Here's the drawing with two shaded views (mm, measured from the low corner). I have some questions. Round coordinates to 2 decimals unless told otherwise and drop trailing zeros. Write each loop counter-clockwise with the first axis right and the second up, starting at its lowest first coordinate (ties: lowest second). Pieces come first, ordered by that corner, then holes. Notation, with made-up numbers: (-24, 86) - (28, 86) arc R15 ccw to (28, 103) - close; hole circle Ø11 at (66.5, 79). An arc over 180 degrees is marked (long way). Return JSON: item names as keys, results as strings. Group by question number.
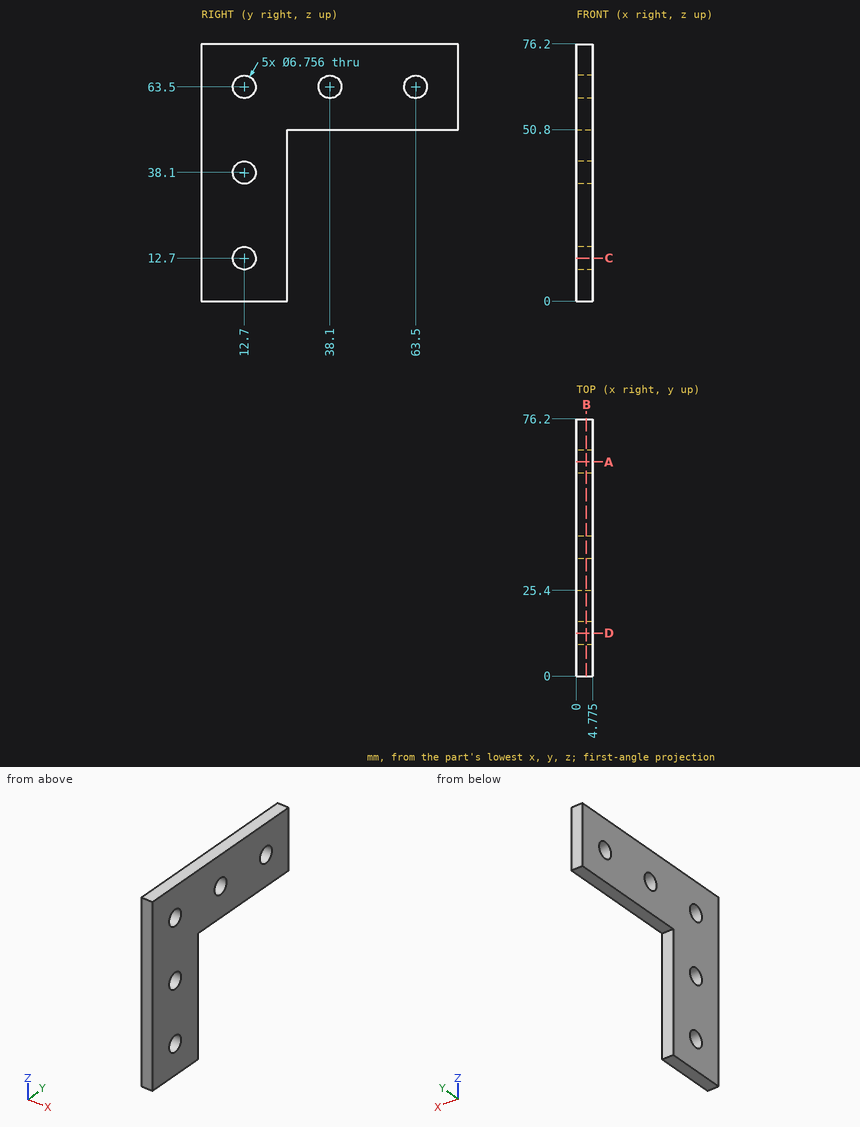
1) Imagine slicing it at A-A (y = 63.5). Please give me the cut outline in (x, z) (1 decimal).
2) Will these pins go through, and if not, where does the flat tip stop? pin 1 Ø1.4 at (x, z) = (1.5, 17.5) entering from +Y; pin 2 Ø6 at (y, z) = (38.1, 63.5) entering from -X; pin 3 Ø2 at (x, y) = (3.5, 47) entering from -Z.
3) I need wall thicknesses on line 1 along Y through (x, z) = (3.45, 63.5); line 2 along Y through (x, z) = (2.3, 47); line 3 along Z through (x, y) = (3.45, 55). Which ranges of each line are inside material? Lowest first, please.
4) Imagine slicing it at C-C (z = 12.7). Please give me the cut outline in (x, y) (1 decimal).
5) Imagine slicing it at B-B (x = 2.95). Please give me the cut outline in (y, z), plus the area to 3 significant figures.
6) Imagine slicing it at D-D (y = 12.7). Please give me the cut outline in (x, z) (1 decimal), plus the area to 3 significant figures.
Results found:
{
 "1": {"outline": "(0, 50.8) - (4.8, 50.8) - (4.8, 60.1) - (0, 60.1) - close; (0, 66.9) - (4.8, 66.9) - (4.8, 76.2) - (0, 76.2) - close"},
 "2": {"pin 1": "stops at y = 25.4", "pin 2": "passes through", "pin 3": "stops at z = 50.8"},
 "3": {"line 1": "y = 0 to 9.32, 16.08 to 34.72, 41.48 to 60.12, 66.88 to 76.2", "line 2": "y = 0 to 25.4", "line 3": "z = 50.8 to 76.2"},
 "4": {"outline": "(0, 0) - (4.8, 0) - (4.8, 9.3) - (0, 9.3) - close; (0, 16.1) - (4.8, 16.1) - (4.8, 25.4) - (0, 25.4) - close"},
 "5": {"outline": "(0, 0) - (25.4, 0) - (25.4, 50.8) - (76.2, 50.8) - (76.2, 76.2) - (0, 76.2) - close; hole circle Ø6.76 at (12.7, 12.7); hole circle Ø6.76 at (12.7, 38.1); hole circle Ø6.76 at (12.7, 63.5); hole circle Ø6.76 at (38.1, 63.5); hole circle Ø6.76 at (63.5, 63.5)", "area": "3,050 mm²"},
 "6": {"outline": "(0, 0) - (4.8, 0) - (4.8, 9.3) - (0, 9.3) - close; (0, 16.1) - (4.8, 16.1) - (4.8, 34.7) - (0, 34.7) - close; (0, 41.5) - (4.8, 41.5) - (4.8, 60.1) - (0, 60.1) - close; (0, 66.9) - (4.8, 66.9) - (4.8, 76.2) - (0, 76.2) - close", "area": "267 mm²"}
}
